The listing builds one solid part. Answer for the finished solid, in the listing's coordinates (mm). A direction names the side the tool comes from. Give positions to 0.01 mm unless a question says otherwise; leave off trailing zeros. Write each loop counter-clockwise with the first axis right and the second up, starting at its lowest first coordinate (ties: lowest second). Pieces come first, ordered by that corner, then holes. Notation, with made-up numbers: (27, 28) -> (79, 28) arc R6 cw to (79, 33) -> close; hole circle Ø11 at (31.25, 17). An arc over 180 degrees is marked (long way). One line per question, with ' | ' between items.
Autodesk Inventor part; units mm, degrees
ref_plane "YZ Plane" through (0, 0, 0) normal (1, 0, 0) x (0, 1, 0)
ref_plane "XZ Plane" through (0, 0, 0) normal (0, 1, 0) x (-1, 0, 0)
ref_plane "XY Plane" through (0, 0, 0) normal (0, 0, 1) x (1, 0, 0)
sketch "Sketch1" plane through (0, 0, 0) normal (0, 1, 0) x (-1, 0, 0)
  line L0 (-43, -78) -> (43, -78)
  line L1 (43, -78) -> (43, 78)
  line L2 (43, 78) -> (-43, 78)
  line L3 (-43, 78) -> (-43, -78)
  point P0 (0, 0)
extrude "Extrusion1" add sketch "Sketch1" along normal blind 3
sketch "Sketch2" plane through (0, 3, 0) normal (0, 1, 0) x (1, 0, 0)
  line L0 (-33, 75) -> (33, 75)
  line L1 (40, 68) -> (40, -68)
  line L2 (33, -75) -> (-33, -75)
  line L3 (-40, -68) -> (-40, 68)
  line L4 (-40, 75) -> (40, -75) construction
  line L5 (40, 75) -> (-40, -75) construction
  line L6 (43, 78) -> (-43, 78)
  line L7 (-43, 78) -> (-43, -78)
  line L8 (-43, -78) -> (43, -78)
  line L9 (43, -78) -> (43, 78)
  line L10 (-40, 75) -> (-33, 75)
  line L11 (-33, 75) -> (-33, 71)
  line L12 (-36, 68) -> (-40, 68)
  line L13 (-40, 68) -> (-40, 75)
  circle A0 centre (-36.5, 71.5) radius 1.5
  arc A1 (-36, 68) -> (-33, 71) centre (-36, 71) ccw
  line L14 (40, 75) -> (-40, -75) construction
  line L15 (33, 75) -> (33, 71)
  line L16 (36, 68) -> (40, 68)
  circle A2 centre (36.5, 71.5) radius 1.5
  arc A3 (33, 71) -> (36, 68) centre (36, 71) ccw
  line L17 (-40, -75) -> (40, 75) construction
  line L18 (-33, -75) -> (-33, -71)
  line L19 (-36, -68) -> (-40, -68)
  circle A4 centre (-36.5, -71.5) radius 1.5
  arc A5 (-33, -71) -> (-36, -68) centre (-36, -71) ccw
  line L20 (36, -68) -> (40, -68)
  arc A6 (36, -68) -> (33, -71) centre (36, -71) ccw
  circle A7 centre (36.5, -71.5) radius 1.5
  line L21 (33, -75) -> (33, -71)
  point P0 (0, 0)
  point P1 (-33, 68)
  point P2 (33, 68)
  point P3 (-33, -68)
  dimension "d5" = 80
  dimension "d6" = 150
  dimension "d7" = 3
  dimension "d42" = 7
  dimension "d43" = 7
  dimension "d45" = 3
  dimension "d46" = 3
extrude "Extrusion2" add sketch "Sketch2" along normal blind 20 contours L11 A1 L12 L13 L10 | L9 L8 L7 L6
fillet "Fillet1" radius 4 4 edges at (-43, 11.5, 78) (43, 11.5, 78) (43, 11.5, -78) (-43, 11.5, -78)
sketch "Sketch3" plane through (0, 3, 0) normal (0, 1, 0) x (1, 0, 0)
  line L0 (-24.5882, 18.801) -> (-24.5882, 15.801)
  line L1 (10, 18.801) -> (10, 15.801)
  line L2 (-24.5882, 18.801) -> (-13.5365, 18.801)
  line L3 (-24.5882, 15.801) -> (-13.5365, 15.801)
  line L4 (10, 18.801) -> (30, 18.801)
  line L5 (10, 15.801) -> (30, 15.801)
  line L6 (30, 18.801) -> (38.3417, 18.801)
  line L7 (30, 15.801) -> (38.3417, 15.801)
  line L8 (38.3417, 18.801) -> (38.3417, 15.801)
  line L9 (-13.5365, 18.801) -> (-13.5365, 15.801)
  point P0 (0, 0)
extrude "Extrusion3" add sketch "Sketch3" along normal blind 10
sketch "Sketch6" plane through (0, 3, 0) normal (0, 1, 0) x (1, 0, 0)
  line L0 (-33, -75) -> (33, -75)
  line L1 (-40, 68) -> (-40, -68)
  line L2 (0, -75) -> (0, -69.5874)
  circle A0 centre (-4.6, -44.9) radius 1.5
  circle A1 centre (-4.6, -44.9) radius 4.5
  circle A2 centre (24.2, -1.9) radius 1.5
  circle A3 centre (24.2, -1.9) radius 4.5
  point P0 (0, 0)
extrude "Extrusion5" add sketch "Sketch6" along normal blind 3
sketch "Sketch7" plane through (-43, 0, -74) normal (-1, 0, 0) x (0, 0, 1)
  line L0 (0, 23) -> (0, 0)
  line L1 (42.5, 8.3188) -> (56, 8.3188)
  line L2 (56, 8.3188) -> (56, 17.1188)
  line L3 (56, 17.1188) -> (42.5, 17.1188)
  line L4 (42.5, 17.1188) -> (42.5, 8.3188)
  line L5 (42.5, 8.3188) -> (56, 17.1188) construction
  line L6 (56, 8.3188) -> (42.5, 17.1188) construction
  point P0 (74, 0)
  dimension "d58" = 13.5
  dimension "d59" = 8.8
extrude "Extrusion6" cut sketch "Sketch7" against normal blind 3
sketch "Sketch8" plane through (-39, 0, 78) normal (0, 0, 1) x (1, 0, 0)
  line L0 (12.7606, 17) -> (23.7606, 17)
  line L1 (25.7606, 15) -> (25.7606, 11)
  line L2 (23.7606, 9) -> (12.7606, 9)
  line L3 (10.7606, 11) -> (10.7606, 15)
  arc A0 (12.7606, 17) -> (10.7606, 15) centre (12.7606, 15) ccw
  arc A1 (25.7606, 15) -> (23.7606, 17) centre (23.7606, 15) ccw
  arc A2 (23.7606, 9) -> (25.7606, 11) centre (23.7606, 11) ccw
  arc A3 (10.7606, 11) -> (12.7606, 9) centre (12.7606, 11) ccw
  line L4 (82, 23) -> (82, 0)
  line L5 (78, 0) -> (0, 0)
  line L6 (71.3066, 0) -> (87.3066, 0) construction
  line L7 (72, 3) -> (72, 23)
  line L8 (72, 11.5) -> (81, 11.5) construction
  line L9 (49, 13) -> (77.3417, 13)
  line L10 (57, 19) -> (67, 19)
  line L11 (69, 17) -> (69, 12)
  line L12 (67, 10) -> (57, 10)
  line L13 (55, 12) -> (55, 17)
  line L14 (55, 19) -> (69, 10) construction
  line L15 (69, 19) -> (55, 10) construction
  line L16 (0, 23) -> (78, 23)
  arc A4 (57, 19) -> (55, 17) centre (57, 17) ccw
  arc A5 (55, 12) -> (57, 10) centre (57, 12) ccw
  arc A6 (69, 17) -> (67, 19) centre (67, 17) ccw
  arc A7 (67, 10) -> (69, 12) centre (67, 12) ccw
  point P0 (39, 0)
  point P1 (25.7606, 9)
  point P2 (25.7606, 17)
  point P3 (10.7606, 9)
  point P4 (69, 13)
  dimension "d68" = 15
  dimension "d69" = 8
  dimension "d70" = 2
  dimension "d98" = 14
  dimension "d99" = 4
  dimension "d100" = 9
  dimension "d101" = 2
  dimension "d102" = 2
  dimension "d103" = 2
  dimension "d104" = 2
  dimension "d105" = 13
  dimension "d106" = 6
extrude "Extrusion7" cut sketch "Sketch8" against normal blind 3
fillet "Fillet3" radius 1.5 8 edges at (-41.8284, 0, 76.8284) (0, 0, 78) (41.8284, 0, 76.8284) (43, 0, 0) (41.8284, 0, -76.8284) (0, 0, -78) (-41.8284, 0, -76.8284) (-43, 0, 0)
properties part number "CASING NEW"
Item 1: Consider line 1 (X direction, y = 19.25, z = -71.5); line 2 (X direction, y = 5.4, z = 44.9); line 3 (Z direction, x = 24.2, y = 4.4). Determine where each line is inside the solid, lowest interval first. Write a range as [from, to].
Answers below:
line 1: [-43, -38], [-35, -33], [33, 35], [38, 43] | line 2: [-43, -40], [-9.1, -6.1], [-3.1, -0.1], [40, 43] | line 3: [-78, -75], [-18.8, -15.8], [-2.6, 0.4], [3.4, 6.4], [75, 78]
Item 2: A tool of negligible diameter and unlimited length cuts with its end or side. For faces 1 (the face through (-41.797, 12.401, -76.859)), 2 (the face through (22.7, 4.48, 1.97)), 3 (the face through (-13.239, 13, 77)), 4 (the face through (-42, 13, -31.5)), from which of +Z, -Z, +X, -X, +Y, -Y can it reach the whole face along a straight path? Write none if from no direction.
Answers below:
face 1: -Z, -X, +Y, -Y | face 2: +Y | face 3: +Z | face 4: -X
Item 3: Determine the mould class of faces 5 (the face through (37, 3, -71)), 6 (the face through (-38, 13, 68)), 7 (the face through (-21, 17, 77)) for opening direction Y: pulls with the +Y half, pulls with the -Y half, needs draft (parallel to the pull), parting line crosses it, or undercut.
Answers below:
face 5: pulls with the +Y half | face 6: needs draft | face 7: undercut
Item 4: Find section B-B (y = 20.5). Write down the section's boundary in (x, z).
Answers below:
outline: (-43, -74) arc R4 ccw to (-39, -78) -> (39, -78) arc R4 ccw to (43, -74) -> (43, 74) arc R4 ccw to (39, 78) -> (-39, 78) arc R4 ccw to (-43, 74) -> close; hole (-40, -68) -> (-36, -68) arc R3 cw to (-33, -71) -> (-33, -75) -> (33, -75) -> (33, -71) arc R3 cw to (36, -68) -> (40, -68) -> (40, 68) -> (36, 68) arc R3 cw to (33, 71) -> (33, 75) -> (-33, 75) -> (-33, 71) arc R3 cw to (-36, 68) -> (-40, 68) -> close; hole circle Ø3 at (-36.5, -71.5); hole circle Ø3 at (-36.5, 71.5); hole circle Ø3 at (36.5, -71.5); hole circle Ø3 at (36.5, 71.5)
Item 5: Flat-ended cylindrical pins translate along their axes: pin 1 (7 mm diameter, centred on x = -5, z = 46, fed in from +Y); pin 2 (6 mm diameter, centred on x = 34, z = 55, fed in from +Y); pin 3 (0.9 mm diameter, centred on x = 18.5, z = -17, fed in from +Y). Find the tip coordinate at first contact, or state that the pin passes through.
Answers below:
pin 1: y = 6 | pin 2: y = 3 | pin 3: y = 13
Item 6: Find section A-A (x = -22). Write down the section's boundary in (y, z), then the cut area to 3 significant figures.
Answers below:
outline: (0, -76.5) arc R1.5 ccw to (1.5, -78) -> (23, -78) -> (23, -75) -> (3, -75) -> (3, -18.8) -> (13, -18.8) -> (13, -15.8) -> (3, -15.8) -> (3, 75) -> (9, 75) -> (9, 78) -> (1.5, 78) arc R1.5 ccw to (0, 76.5) -> close; (17, 75) -> (23, 75) -> (23, 78) -> (17, 78) -> close | area: 593 mm²
Item 7: Find section D-D (z = 44.9). Write down the section's boundary in (x, y).
Answers below:
outline: (-43, 1.5) arc R1.5 ccw to (-41.5, 0) -> (41.5, 0) arc R1.5 ccw to (43, 1.5) -> (43, 23) -> (40, 23) -> (40, 3) -> (-0.1, 3) -> (-0.1, 6) -> (-3.1, 6) -> (-3.1, 3) -> (-6.1, 3) -> (-6.1, 6) -> (-9.1, 6) -> (-9.1, 3) -> (-40, 3) -> (-40, 23) -> (-43, 23) -> close
Item 8: Find section C-C (x = -4.6). Write down the section's boundary in (y, z).
Answers below:
outline: (0, -76.5) arc R1.5 ccw to (1.5, -78) -> (23, -78) -> (23, -75) -> (3, -75) -> (3, 40.4) -> (6, 40.4) -> (6, 43.4) -> (3, 43.4) -> (3, 46.4) -> (6, 46.4) -> (6, 49.4) -> (3, 49.4) -> (3, 75) -> (23, 75) -> (23, 78) -> (1.5, 78) arc R1.5 ccw to (0, 76.5) -> close
